Part model, mm, in its own coordinate system. Face numbers are marked on the shaded views. A direction names the side the tool comes from. Coordinates: 2 decimals unless noted, no trailing zeros. Loops run counter-clockwise (first coordinate to the right, second up) from the corner with the lowest first, then second, coordinate; pieces in that order, holes last. Notation, with made-up numbers: (-37, 64.25) -> (-27, 64.25) arc R9 ccw to (-27, 68.25) -> close; hole circle Ø10 at (52.5, -2). An arc over 180 degrees is marked (long way). One line per item, written item: value. Start each with the question number.
Solid Edge part; units mm, degrees
sketch "Sketch1" plane through (0, 0, 0) normal (0, -1, 0) x (1, 0, 0)
  line L0 (1.5, 0) -> (3, 1.5)
  line L1 (3, 1.5) -> (3, 1.7)
  line L2 (3, 1.7) -> (0, 1.7)
  line L3 (0, 1.7) -> (0, -23.3)
  line L4 (0, -23.3) -> (1.1935, -23.3)
  line L5 (1.1935, -23.3) -> (1.5, -22.9935)
  line L6 (1.5, -22.9935) -> (1.5, -11.3)
  line L7 (1.5, -11.3) -> (1.1935, -11.3)
  line L8 (1.1935, -11.3) -> (1.1935, -11.29)
  line L9 (1.1935, -11.29) -> (1.5, -11.29)
  line L10 (1.5, -11.29) -> (1.5, 0)
  dimension "D1" = 1.5
  dimension "D2" = 1.1935
revolve "RevolvedProtrusion1" add sketch "Sketch1" angle 360 about axis through (0, 0, 54) along (0, 0, -1)
sketch "Sketch2" plane through (0, 0, 0) normal (0, -1, 0) x (1, 0, 0)
  arc A0 (-1, 0.5) -> (0, 0) centre (0, 1.25) ccw
  line L0 (0, 0.5) -> (0, 0)
  line L1 (-1, 0.5) -> (0, 0.5)
revolve "RevolvedCutout1" cut sketch "Sketch2" angle 360 about axis through (0, 0, 54) along (0, 0, -1)
sketch "Sketch3" plane through (0, 0, 1.7) normal (0, 0, 1) x (0, -1, 0)
  line L0 (-1.1547, 0) -> (-0.5774, 1)
  line L1 (-0.5774, 1) -> (0.5774, 1)
  line L2 (0.5774, 1) -> (1.1547, 0)
  line L3 (1.1547, 0) -> (0.5774, -1)
  line L4 (0.5774, -1) -> (-0.5774, -1)
  line L5 (-0.5774, -1) -> (-1.1547, 0)
extrude "Cutout1" cut sketch "Sketch3" against normal blind 1.2
cosmetic_thread "Thread1"
sketch "Sketch4" plane through (0, 0, 0) normal (1, 0, 0) x (0, 1, 0)
  line L0 (-1.15, 1.7) -> (0, 1.036)
revolve "RevolvedCutout2" cut sketch "Sketch4" angle 360 about axis through (0, 0, -57) along (0, 0, 1) material side at (0, -0.55, 1.4113)
fillet "Round1" radius 0.1 1 edges at (-1.5, 0, 0)
properties material "Stahl"
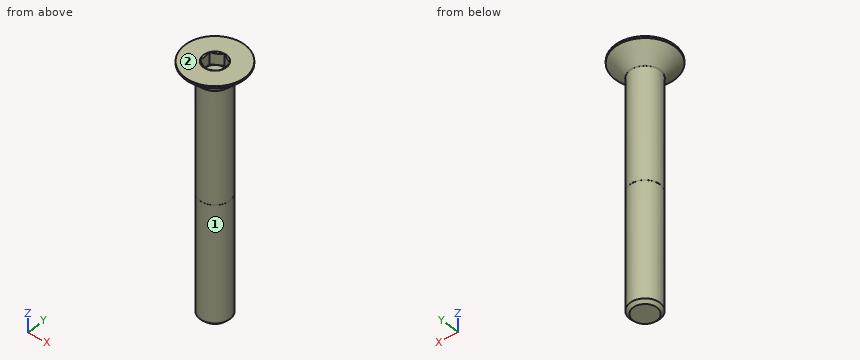
1) Probe line 1 (Y direction, x = -1, z = -21.25); line 2 (Y direction, x = 1.25, z = -0.25); line 3 (Z direction, x = 1.75, y = 2). List the from-to ranges inside material, lowest first. Write a range as from..to.
2) Slice it at A-A (z = -7.25). Give the cut face in (x, y).
3) Pin check, flat tips, straight feed: pin 1 Ø2 at (y, z) = (1.5, -8) entering from -X; pin 2 Ø1.5 at (x, y) = (-1.5, 2) entering from -Z; pin 3 Ø2 at (x, z) = (-0.5, -6) entering from +Y; pin 4 Ø3 at (x, y) = (-1, 1) entering from -Z. Stop position of each tip, or through.
4) Tool access for the marked faces 1 and 2: list every direction of +Z, -Z, +X, -X, +Y, -Y with a clear straight run to the whole face (end or side of a thin tool).
Check sheet entries:
1. line 1: y = -1.12..1.12
1. line 2: y = -0.83..0.83
1. line 3: z = 1.16..1.7
2. outline: circle Ø3 at (0, 0)
3. pin 1: stops at x = -1.41
3. pin 2: stops at z = 0.25
3. pin 3: stops at y = 1.5
3. pin 4: stops at z = -23.3
4. face 1: -Z
4. face 2: +Z, +X, -X, +Y, -Y
